For this review, take the finished solid that the model builds, in its own axes (mm). Face numbers are marked on the shaded views. A direction names the side the tool comes from. Coordinates: 2 decimals unless noted, no trailing zeros. Write each loop counter-clockwise with the first axis right and the second up, starting at its lowest first coordinate (ties: lowest second). Pieces come first, ordered by that corner, then holes. Notation, with made-up numbers: (-30.5, -27) - (-25.5, -27) arc R17 ccw to (-25.5, -14) - close; hole circle Ø3 at (-29.75, -12.5). An arc over 180 degrees is marked (long way). Write each question's results on one line, items separated by ' | '.
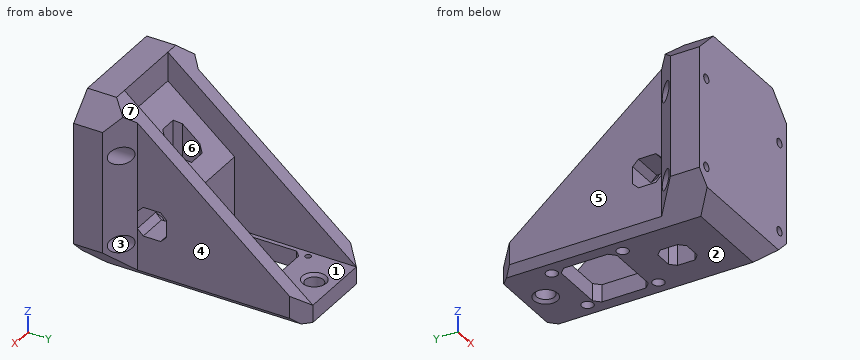
from build123d import *

# Parameters (mm, degrees)
SKETCH1_W           = 50
SKETCH1_H           = 60
BOSS_EXTRUDE1_DEPTH = 10
SKETCH2_R           = 1.5
CUT_EXTRUDE1_DEPTH  = 6
CUT_EXTRUDE2_REACH  = 41.509
SKETCH3_R           = 3
SKETCH5_W           = 25
SKETCH5_H           = 6
BOSS_EXTRUDE3_DEPTH = 65
CUT_EXTRUDE3_REACH  = 101.247
SKETCH6_W           = 22
SKETCH6_H           = 19.25
SKETCH7_R           = 1
CUT_EXTRUDE4_DEPTH  = 2.5
CUT_EXTRUDE5_REACH  = 99.171
SKETCH8_R           = 2
BOSS_EXTRUDE4_DEPTH = 5
CHAMFER1_SIZE       = 7.5
CHAMFER2_SIZE       = 10
CHAMFER4_SIZE       = 5.5
CHAMFER5_SIZE       = 5
CHAMFER7_SIZE       = 2
CUT_EXTRUDE6_REACH  = 101.247
SKETCH10_R          = 3.1
CHAMFER8_SIZE       = 1
BOSS_EXTRUDE5_REACH = 91.058
CHAMFER9_SIZE       = 8
CUT_EXTRUDE7_REACH  = 101.247
SKETCH12_W          = 10
SKETCH12_H          = 10
CUT_EXTRUDE9_REACH  = 88.168
SKETCH14_W          = 10
SKETCH14_H          = 10
CHAMFER11_SIZE      = 2


with BuildPart() as part:
    # Sketch1 → Boss-Extrude1 (new body)
    with BuildSketch(Plane(origin=(0, 0, 0), x_dir=(1, 0, 0), z_dir=(0, 1, 0))):
        Rectangle(SKETCH1_W, SKETCH1_H)
    extrude(amount=BOSS_EXTRUDE1_DEPTH)

    # Sketch2 → Cut-Extrude1 (cut)
    with BuildSketch(Plane(origin=(0, 0, 0), x_dir=(1, 0, 0), z_dir=(0, 1, 0))):
        with Locations(Location((-21, 17.7, 0), (0, 0, 270))):
            Circle(SKETCH2_R)
        with Locations(Location((-21, -13, 0), (0, 0, 270))):
            Circle(SKETCH2_R)
        with Locations(Location((21, 17.7, 0), (0, 0, 270))):
            Circle(SKETCH2_R)
        with Locations(Location((21, -13, 0), (0, 0, 270))):
            Circle(SKETCH2_R)
    extrude(amount=CUT_EXTRUDE1_DEPTH, mode=Mode.SUBTRACT)

    # Sketch3 → Cut-Extrude2 (cut, up to next)
    with BuildSketch(Plane.XZ.offset(-6), mode=Mode.PRIVATE) as cut_extrude2_sk1:
        with Locations(Location((-21, 13, 0), (0, 0, 270))):
            Circle(SKETCH3_R)
    cut_extrude2_tool1 = extrude(cut_extrude2_sk1.sketch, amount=-CUT_EXTRUDE2_REACH, mode=Mode.PRIVATE) & part.part
    # Sketch3 → Cut-Extrude2 (cut, up to next)
    with BuildSketch(Plane.XZ.offset(-6), mode=Mode.PRIVATE) as cut_extrude2_sk2:
        with Locations(Location((21, 13, 0), (0, 0, 270))):
            Circle(SKETCH3_R)
    cut_extrude2_tool2 = extrude(cut_extrude2_sk2.sketch, amount=-CUT_EXTRUDE2_REACH, mode=Mode.PRIVATE) & part.part
    # Sketch3 → Cut-Extrude2 (cut, up to next)
    with BuildSketch(Plane.XZ.offset(-6), mode=Mode.PRIVATE) as cut_extrude2_sk3:
        with Locations(Location((21, -17.7, 0), (0, 0, 270))):
            Circle(SKETCH3_R)
    cut_extrude2_tool3 = extrude(cut_extrude2_sk3.sketch, amount=-CUT_EXTRUDE2_REACH, mode=Mode.PRIVATE) & part.part
    # Sketch3 → Cut-Extrude2 (cut, up to next)
    with BuildSketch(Plane.XZ.offset(-6), mode=Mode.PRIVATE) as cut_extrude2_sk4:
        with Locations(Location((-21, -17.7, 0), (0, 0, 270))):
            Circle(SKETCH3_R)
    cut_extrude2_tool4 = extrude(cut_extrude2_sk4.sketch, amount=-CUT_EXTRUDE2_REACH, mode=Mode.PRIVATE) & part.part
    add(cut_extrude2_tool1.solids().sort_by_distance((-21, 6, 13))[0], mode=Mode.SUBTRACT)
    add(cut_extrude2_tool2.solids().sort_by_distance((21, 6, 13))[0], mode=Mode.SUBTRACT)
    add(cut_extrude2_tool3.solids().sort_by_distance((21, 6, -17.7))[0], mode=Mode.SUBTRACT)
    add(cut_extrude2_tool4.solids().sort_by_distance((-21, 6, -17.7))[0], mode=Mode.SUBTRACT)

    # Sketch5 → Boss-Extrude3 (add)
    with BuildSketch(Plane(origin=(0, 10, 0), x_dir=(1, 0, 0), z_dir=(0, 1, 0))):
        with Locations((0, 27)):
            Rectangle(SKETCH5_W, SKETCH5_H)
    extrude(amount=BOSS_EXTRUDE3_DEPTH)

    # Sketch6 → Cut-Extrude3 (cut, up to next)
    with BuildSketch(Plane(origin=(0, 0, -30), x_dir=(-1, 0, 0), z_dir=(0, 0, -1)), mode=Mode.PRIVATE) as cut_extrude3_sk1:
        with Locations((0, 47.625)):
            Rectangle(SKETCH6_W, SKETCH6_H)
    cut_extrude3_tool1 = extrude(cut_extrude3_sk1.sketch, amount=-CUT_EXTRUDE3_REACH, mode=Mode.PRIVATE) & part.part
    add(cut_extrude3_tool1.solids().sort_by_distance((0, 47.625, -30))[0], mode=Mode.SUBTRACT)

    # Sketch7 → Cut-Extrude4 (cut)
    with BuildSketch(Plane.XY.offset(-24)):
        with Locations((10.25, 35.25)):
            Circle(SKETCH7_R)
        with Locations((-10.25, 35.25)):
            Circle(SKETCH7_R)
        with Locations((-10.25, 59.7)):
            Circle(SKETCH7_R)
        with Locations((10.25, 59.7)):
            Circle(SKETCH7_R)
    extrude(amount=-CUT_EXTRUDE4_DEPTH, mode=Mode.SUBTRACT)

    # Sketch8 → Cut-Extrude5 (cut, up to next)
    with BuildSketch(Plane.XY.offset(-26.5), mode=Mode.PRIVATE) as cut_extrude5_sk1:
        with Locations((-10.25, 59.7)):
            Circle(SKETCH8_R)
    cut_extrude5_tool1 = extrude(cut_extrude5_sk1.sketch, amount=-CUT_EXTRUDE5_REACH, mode=Mode.PRIVATE) & part.part
    # Sketch8 → Cut-Extrude5 (cut, up to next)
    with BuildSketch(Plane.XY.offset(-26.5), mode=Mode.PRIVATE) as cut_extrude5_sk2:
        with Locations((10.25, 59.7)):
            Circle(SKETCH8_R)
    cut_extrude5_tool2 = extrude(cut_extrude5_sk2.sketch, amount=-CUT_EXTRUDE5_REACH, mode=Mode.PRIVATE) & part.part
    # Sketch8 → Cut-Extrude5 (cut, up to next)
    with BuildSketch(Plane.XY.offset(-26.5), mode=Mode.PRIVATE) as cut_extrude5_sk3:
        with Locations((10.25, 35.25)):
            Circle(SKETCH8_R)
    cut_extrude5_tool3 = extrude(cut_extrude5_sk3.sketch, amount=-CUT_EXTRUDE5_REACH, mode=Mode.PRIVATE) & part.part
    # Sketch8 → Cut-Extrude5 (cut, up to next)
    with BuildSketch(Plane.XY.offset(-26.5), mode=Mode.PRIVATE) as cut_extrude5_sk4:
        with Locations((-10.25, 35.25)):
            Circle(SKETCH8_R)
    cut_extrude5_tool4 = extrude(cut_extrude5_sk4.sketch, amount=-CUT_EXTRUDE5_REACH, mode=Mode.PRIVATE) & part.part
    add(cut_extrude5_tool1.solids().sort_by_distance((-10.25, 59.7, -26.5))[0], mode=Mode.SUBTRACT)
    add(cut_extrude5_tool2.solids().sort_by_distance((10.25, 59.7, -26.5))[0], mode=Mode.SUBTRACT)
    add(cut_extrude5_tool3.solids().sort_by_distance((10.25, 35.25, -26.5))[0], mode=Mode.SUBTRACT)
    add(cut_extrude5_tool4.solids().sort_by_distance((-10.25, 35.25, -26.5))[0], mode=Mode.SUBTRACT)

    # Sketch9 → Boss-Extrude4 (add)
    with BuildSketch(Plane(origin=(12.5, 0, 0), x_dir=(0, 0, -1), z_dir=(1, 0, 0))):
        Polygon((30, 75), (24, 75), (-30, 10), (30, 10), align=None)
    boss_extrude4 = extrude(amount=BOSS_EXTRUDE4_DEPTH)

    # Mirror1: Boss-Extrude4 across plane
    add(boss_extrude4.mirror(Plane(origin=(0, 0, 0), x_dir=(0, 0, 1), z_dir=(1, 0, 0))))

    # Chamfer1
    # the kernel refuses this chamfer: 7.5 mm, written as the material it adds along each edge
    with BuildSketch(Plane(origin=(17.5, 10, 30), x_dir=(0.9996219169112968, -0.02749587661058632, 0), z_dir=(0, 0, -1))) as chamfer1_piece_1_section:
        Polygon((CHAMFER1_SIZE * 0.999621916911, -CHAMFER1_SIZE * 0.0274958766106), (-CHAMFER1_SIZE * 0.0274958766106, -CHAMFER1_SIZE * 0.999621916911), (0, 0), align=None)
    chamfer1_piece_1 = extrude(amount=60, mode=Mode.PRIVATE)
    chamfer1_piece_1 = split(chamfer1_piece_1, bisect_by=Plane(origin=(19.919237696, 26.599778663, 16.209414649), z_dir=(0, -0.6390196945354667, -0.7691903730519506)), keep=Keep.TOP, mode=Mode.PRIVATE)
    chamfer1_piece_1 = chamfer1_piece_1 - Plane(origin=(21, 12.462621572, -17.7), x_dir=(0, 0, -1), z_dir=(0, -1, 0)) * Cylinder(3, 150, mode=Mode.PRIVATE)
    chamfer1_piece_1 = chamfer1_piece_1 - Plane(origin=(21, 12.462621572, 13), x_dir=(0, 0, -1), z_dir=(0, -1, 0)) * Cylinder(3, 150, mode=Mode.PRIVATE)
    chamfer1_piece_1 = split(chamfer1_piece_1, bisect_by=Plane(origin=(25, 12.462621572, -0.807533702), z_dir=(-1, 0, 0)), keep=Keep.TOP, mode=Mode.PRIVATE)
    add(chamfer1_piece_1)
    with BuildSketch(Plane(origin=(-17.5, 10, 30), x_dir=(0.02749587661058632, 0.9996219169112968, 0), z_dir=(0, 0, -1))) as chamfer1_piece_2_section:
        Polygon((CHAMFER1_SIZE * 0.999621916911, -CHAMFER1_SIZE * 0.0274958766106), (-CHAMFER1_SIZE * 0.0274958766106, -CHAMFER1_SIZE * 0.999621916911), (0, 0), align=None)
    chamfer1_piece_2 = extrude(amount=60, mode=Mode.PRIVATE)
    chamfer1_piece_2 = split(chamfer1_piece_2, bisect_by=Plane(origin=(-19.919241024, 26.599776134, 16.209416751), z_dir=(0, -0.6390196945354667, -0.7691903730519506)), keep=Keep.TOP, mode=Mode.PRIVATE)
    chamfer1_piece_2 = chamfer1_piece_2 - Plane(origin=(-21, 12.462621922, -17.7), x_dir=(0, 0, -1), z_dir=(0, -1, 0)) * Cylinder(3, 150, mode=Mode.PRIVATE)
    chamfer1_piece_2 = chamfer1_piece_2 - Plane(origin=(-21, 12.462621922, 13), x_dir=(0, 0, -1), z_dir=(0, -1, 0)) * Cylinder(3, 150, mode=Mode.PRIVATE)
    chamfer1_piece_2 = split(chamfer1_piece_2, bisect_by=Plane(origin=(-25, 12.462621922, -0.807528134), z_dir=(1, 0, 0)), keep=Keep.TOP, mode=Mode.PRIVATE)
    add(chamfer1_piece_2)

    # Chamfer2
    chamfer2_edges = [part.edges().sort_by_distance(p)[0] for p in [
        (-25, 5, -30),
        (25, 5, -30),
    ]]
    chamfer(chamfer2_edges, length=CHAMFER2_SIZE)

    # Chamfer4
    chamfer4_edges = [part.edges().sort_by_distance(p)[0] for p in [
        (0, 0, -30),
    ]]
    chamfer(chamfer4_edges, length=CHAMFER4_SIZE)

    # Chamfer5
    chamfer5_edges = [part.edges().sort_by_distance(p)[0] for p in [
        (17.5, 75, -25.75),
        (-17.5, 75, -25.75),
    ]]
    chamfer(chamfer5_edges, length=CHAMFER5_SIZE)

    # Chamfer7
    chamfer7_edges = [part.edges().sort_by_distance(p)[0] for p in [
        (-11, 57.25, -27),
        (-11, 38, -27),
        (11, 38, -27),
        (11, 57.25, -27),
    ]]
    chamfer(chamfer7_edges, length=CHAMFER7_SIZE)

    # Sketch10 → Cut-Extrude6 (cut, up to next)
    with BuildSketch(Plane(origin=(0, 0, -30), x_dir=(-1, 0, 0), z_dir=(0, 0, -1)), mode=Mode.PRIVATE) as cut_extrude6_sk1:
        with Locations((0, 68)):
            Circle(SKETCH10_R)
    cut_extrude6_tool1 = extrude(cut_extrude6_sk1.sketch, amount=-CUT_EXTRUDE6_REACH, mode=Mode.PRIVATE) & part.part
    add(cut_extrude6_tool1.solids().sort_by_distance((0, 68, -30))[0], mode=Mode.SUBTRACT)

    # Chamfer8
    chamfer8_edges = [part.edges().sort_by_distance(p)[0] for p in [
        (3.1, 68, -30),
        (3.1, 68, -24),
    ]]
    chamfer(chamfer8_edges, length=CHAMFER8_SIZE)

    # Sketch11 → Boss-Extrude5 (add, up to next)
    with BuildSketch(Plane(origin=(-12.5, 0, 0), x_dir=(0, 0, -1), z_dir=(1, 0, 0)), mode=Mode.PRIVATE) as boss_extrude5_sk1:
        Polygon((-20, 10), (24, 10), (24, 33), (-0.892307692, 33), align=None)
    boss_extrude5_tool1 = extrude(boss_extrude5_sk1.sketch, amount=BOSS_EXTRUDE5_REACH, mode=Mode.PRIVATE) - part.part
    add(boss_extrude5_tool1.solids().sort_by_distance((-12.5, 20.436802, -6.335287))[0])

    # Chamfer9
    chamfer9_edges = [part.edges().sort_by_distance(p)[0] for p in [
        (25, 5, 30),
        (-25, 5, 30),
    ]]
    chamfer(chamfer9_edges, length=CHAMFER9_SIZE)

    # Cut-Extrude7: up to this plane
    cut_extrude7_end = Plane(origin=(25.002, 33, 0.892307692), z_dir=(0, -0.6390196945354668, -0.7691903730519506))
    # Sketch12 → Cut-Extrude7 (cut, up to the surface)
    with BuildSketch(Plane(origin=(0, 0, -30), x_dir=(-1, 0, 0), z_dir=(0, 0, -1)), mode=Mode.PRIVATE) as cut_extrude7_sk1:
        with Locations((0, 22.5)):
            Rectangle(SKETCH12_W, SKETCH12_H)
    cut_extrude7_tool1 = split(extrude(cut_extrude7_sk1.sketch, amount=-CUT_EXTRUDE7_REACH, mode=Mode.PRIVATE), bisect_by=cut_extrude7_end, keep=Keep.BOTH, mode=Mode.PRIVATE)
    add(cut_extrude7_tool1.solids().sort_by_distance((0, 22.5, -30))[0], mode=Mode.SUBTRACT)

    # Sketch14 → Cut-Extrude9 (cut, up to next)
    with BuildSketch(Plane(origin=(-5, 0, 0), x_dir=(0, 0, -1), z_dir=(1, 0, 0)), mode=Mode.PRIVATE) as cut_extrude9_sk1:
        with Locations((10, 22.5)):
            Rectangle(SKETCH14_W, SKETCH14_H)
    cut_extrude9_tool1 = extrude(cut_extrude9_sk1.sketch, amount=-CUT_EXTRUDE9_REACH, mode=Mode.PRIVATE) & part.part
    cut_extrude9 = cut_extrude9_tool1.solids().sort_by_distance((-5, 22.5, -10))[0]
    add(cut_extrude9, mode=Mode.SUBTRACT)

    # Mirror2: Cut-Extrude9 across plane
    add(cut_extrude9.mirror(Plane(origin=(0, 0, 0), x_dir=(0, 0, 1), z_dir=(1, 0, 0))), mode=Mode.SUBTRACT)

    # Chamfer11
    chamfer11_edges = [part.edges().sort_by_distance(p)[0] for p in [
        (-5, 17.5, 4.384615385),
        (5, 17.5, 4.384615385),
        (5, 27.5, 0.230769231),
        (-5, 27.5, 0.230769231),
        (-5, 17.5, -22.5),
        (-5, 27.5, -22.5),
        (-11.25, 17.5, -15),
        (-11.25, 27.5, -15),
        (-11.25, 17.5, -5),
        (-11.25, 27.5, -5),
        (-5, 22.5, -15),
        (-5, 22.5, -5),
        (5, 27.5, -22.5),
        (5, 17.5, -22.5),
        (11.25, 17.5, -5),
        (11.25, 17.5, -15),
        (5, 22.5, -15),
        (11.25, 27.5, -15),
        (11.25, 27.5, -5),
        (5, 22.5, -5),
    ]]
    chamfer(chamfer11_edges, length=CHAMFER11_SIZE)


solid = part.part
Q1. Take a section at A-A on x = 0. State the section outline as (y, z) points, plus the area to 3 significant figures.
Results found:
outline: (0, -24.5) - (5.5, -30) - (17.5, -30) - (17.5, 13.77) - (10, 20) - (10, 30) - (0, 30) - close; (27.5, -30) - (38, -30) - (38, -24) - (33, -24) - (33, 0.89) - (27.5, 5.46) - close; (57.25, -30) - (63.9, -30) - (64.9, -29) - (64.9, -25) - (63.9, -24) - (57.25, -24) - close; (71.1, -29) - (72.1, -30) - (75, -30) - (75, -24) - (72.1, -24) - (71.1, -25) - close | area: 1,220 mm2
Q2. Wall thickness on line 1 along X through (y, z) = (57, -21); line 2 along X through (y, z) = (3.25, -17.7); line 3 along Y through (x, z) = (-8, -12): over which ranges is each line inside the solid? List them lowest first. Write a range as from..to.
Results found:
line 1: -17.5..-12.5, 12.5..17.5 | line 2: -25..-22.5, -19.5..19.5, 22.5..25 | line 3: 0..17.5, 27.5..33
Q3. Take a section at D-D on x = 13.5. State the section outline as (y, z) points.
Results found:
outline: (0, -24.5) - (5.5, -30) - (74, -30) - (74, -23.17) - (10, 30) - (0, 30) - close; hole (17.5, -13) - (19.5, -15) - (25.5, -15) - (27.5, -13) - (27.5, -7) - (25.5, -5) - (19.5, -5) - (17.5, -7) - close
Q4. For pin 1 (3 mm diameter, centred on y = 51, z = -2, fed in from +X); pin 2 (1.8 mm diameter, centred on y = 22.5, z = 2, fed in from -X); pin 3 (1.8 mm diameter, centred on x = 13, y = 23.5, fed in from +Z); pin 4 (3 mm diameter, centred on y = 22, z = 3.5, fed in from +X), all flat-tipped, find the tip position at first contact; note any pin that passes through.
Results found:
pin 1: through | pin 2: x = -17.5 | pin 3: z = 19.53 | pin 4: x = 17.5
Q5. For the marked faces 1, 2, 3 and 4, list the 3-axis set-ups (+Z, -Z, +X, -X, +Y, -Y) from which the entire face can be reached by the end or side of a thin tool; tool diameter is ignored.
Results found:
face 1: +Z, +Y | face 2: -Z, +X, -X, +Y, -Y | face 3: +Y | face 4: +Z, -Z, +X, +Y
Q6. Mouldability with a two-part tool opening along X and no side actions: class the marked faces 5, 6 and 7 as pulls with the +X half, pulls with the -X half, needs draft (parallel to the pull), parting line crosses it, or undercut.
Results found:
face 5: pulls with the -X half | face 6: undercut | face 7: needs draft
Q7. Take a section at B-B on y = 68. State the section outline as (x, z) points, plus the area to 3 significant figures.
Results found:
outline: (-17.5, -27.5) - (-15, -30) - (-4.1, -30) - (-3.1, -29) - (-3.1, -25) - (-4.1, -24) - (-12.5, -24) - (-12.5, -18.18) - (-17.5, -18.18) - close; (3.1, -29) - (4.1, -30) - (15, -30) - (17.5, -27.5) - (17.5, -18.18) - (12.5, -18.18) - (12.5, -24) - (4.1, -24) - (3.1, -25) - close | area: 223 mm2
Q8. Take a section at C-C on y = 35.25. State the section outline as (x, z) points.
Results found:
outline: (-17.5, -27.5) - (-15, -30) - (-12.25, -30) - (-12.25, -26.5) - (-11.25, -26.5) - (-11.25, -24) - (-12.5, -24) - (-12.5, 9.02) - (-17.5, 9.02) - close; (-9.25, -26.5) - (-8.25, -26.5) - (-8.25, -30) - (8.25, -30) - (8.25, -26.5) - (9.25, -26.5) - (9.25, -24) - (-9.25, -24) - close; (11.25, -26.5) - (12.25, -26.5) - (12.25, -30) - (15, -30) - (17.5, -27.5) - (17.5, 9.02) - (12.5, 9.02) - (12.5, -24) - (11.25, -24) - close
